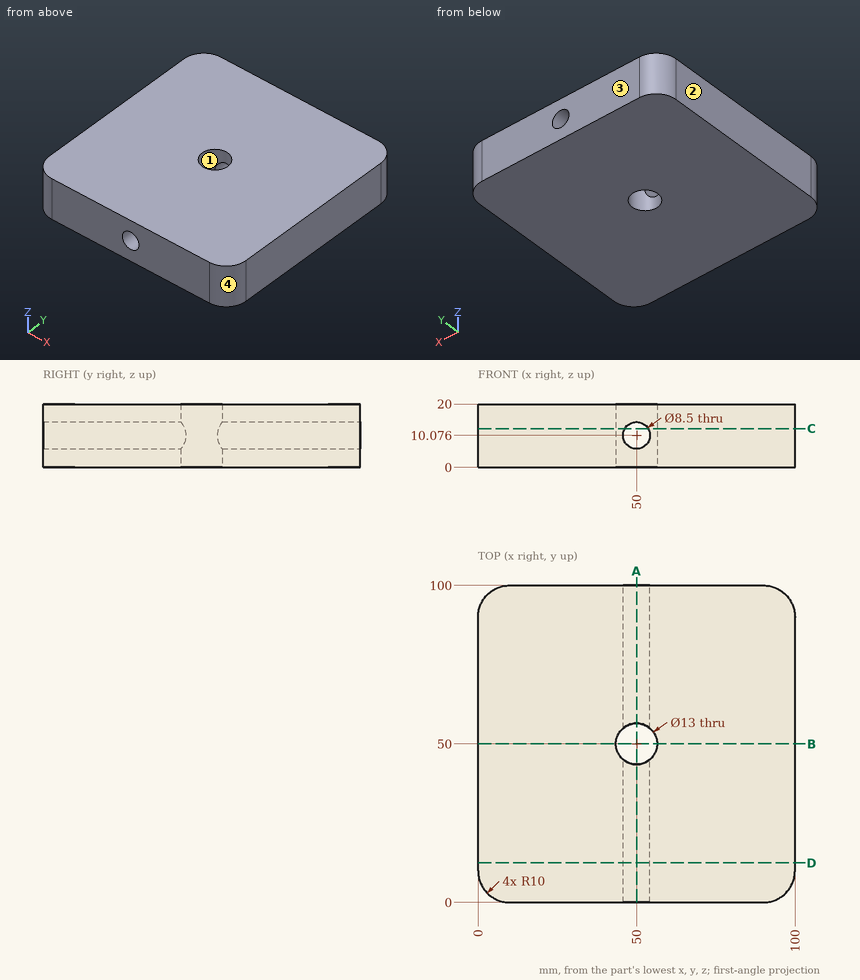
Verification items for this drawing (mm, ordinates from the low corner). Coordinates: 2 decimals unless noted, no trailing zeros. Loops run counter-clockwise (first coordinate to the right, second up) from the corner with the lowest first, then second, coordinate; pieces in that order, holes last.
Item 1: Go/stop test with a flat-tipped pin: pin 1 Ø1.5 at (y, z) = (80.5, 11.5) entering from -X. Record where the tip stops, or that it passes through.
Item 2: Sectioned sample at C-C, the plane z = 12.25. Record the boundary of the cut face in (x, y).
Item 3: Release check for a two-part mould opening along X. For the marked faces 1, 2, 3 and 4 record: released by +X, released by -X, zero draft, split by the parting line, or undercut.
Item 4: Sectioned sample at D-D, the plane y = 12.5. Record the boundary of the cut face in (x, z).
Item 5: Sectioned sample at B-B, the plane y = 50. Record the boundary of the cut face in (x, z).
Item 6: Thickness scan on line 1 (Z direction, x = 50, y = 9.5); line 2 (X direction, y = 45.5, z = 7.25); line 3 (X direction, y = 91, z = 7.5). Record the ranges inside material, lowest first.
Item 7: Sectioned sample at A-A, the plane x = 50. Record the boundary of the cut face in (y, z).
Check result:
1. pin 1: stops at x = 0
2. outline: (0, 10) arc R10 ccw to (10, 0) - (46.35, 0) - (46.35, 44.62) arc R6.5 cw to (46.35, 55.38) - (46.35, 100) - (10, 100) arc R10 ccw to (0, 90) - close; (53.65, 0) - (90, 0) arc R10 ccw to (100, 10) - (100, 90) arc R10 ccw to (90, 100) - (53.65, 100) - (53.65, 55.38) arc R6.5 cw to (53.65, 44.62) - close
3. face 1: undercut
3. face 2: released by -X
3. face 3: zero draft
3. face 4: released by +X
4. outline: (0, 0) - (100, 0) - (100, 20) - (0, 20) - close; hole circle Ø8.5 at (50, 10.08)
5. outline: (0, 0) - (43.5, 0) - (43.5, 20) - (0, 20) - close; (56.5, 0) - (100, 0) - (100, 20) - (56.5, 20) - close
6. line 1: z = 0 to 5.83, 14.33 to 20
6. line 2: x = 0 to 45.31, 54.69 to 100
6. line 3: x = 0.05 to 46.62, 53.38 to 99.95
7. outline: (0, 0) - (43.5, 0) - (43.5, 5.83) - (0, 5.83) - close; (0, 14.33) - (43.5, 14.33) - (43.5, 20) - (0, 20) - close; (56.5, 0) - (100, 0) - (100, 5.83) - (56.5, 5.83) - close; (56.5, 14.33) - (100, 14.33) - (100, 20) - (56.5, 20) - close
